```python
from build123d import *

# Parameters (mm, degrees)
SKETCH1_R           = 1.55
BOSS_EXTRUDE1_DEPTH = 5.8


with BuildPart() as part:
    # Sketch1 → Boss-Extrude1 (new body)
    with BuildSketch(Plane.XY):
        Polygon((-213.609090909, 31.65), (-213.609090909, 38.5), (-188.609090909, 38.5), (-188.609090909, 31.65), (-163.609090909, 31.65), (-163.609090909, 38.5), (-138.609090909, 38.5), (-138.609090909, 31.65), (-113.609090909, 31.65), (-113.609090909, 38.5), (-88.609090909, 38.5), (-88.609090909, 31.65), (-63.609090909, 31.65), (-63.609090909, 38.5), (-38.609090909, 38.5), (-38.609090909, 31.65), (-13.609090909, 31.65), (-13.609090909, 38.5), (11.390909091, 38.5), (11.390909091, 31.65), (36.390909091, 31.65), (36.390909091, 38.5), (61.390909091, 38.5), (61.390909091, 31.65), (86.390909091, 31.65), (86.390909091, 38.5), (111.390909091, 38.5), (111.390909091, 31.65), (136.390909091, 31.65), (136.390909091, 38.5), (161.390909091, 38.5), (161.390909091, 31.65), (186.390909091, 31.65), (186.390909091, 38.5), (211.390909091, 38.5), (211.390909091, 31.65), (236.390909091, 31.65), (236.390909091, 38.5), (261.390909091, 38.5), (261.390909091, 31.65), (274.040909091, 31.65), (274.040909091, 23.35), (283.890909091, 23.35), (283.890909091, 5.45), (274.040909091, 5.45), (274.040909091, -11.15), (283.890909091, -11.15), (283.890909091, -29.05), (274.040909091, -29.05), (274.040909091, -37.35), (261.390909091, -37.35), (261.390909091, -43.15), (236.390909091, -43.15), (236.390909091, -37.35), (211.390909091, -37.35), (211.390909091, -43.15), (186.390909091, -43.15), (186.390909091, -37.35), (161.390909091, -37.35), (161.390909091, -43.15), (136.390909091, -43.15), (136.390909091, -37.35), (111.390909091, -37.35), (111.390909091, -43.15), (86.390909091, -43.15), (86.390909091, -37.35), (61.390909091, -37.35), (61.390909091, -43.15), (36.390909091, -43.15), (36.390909091, -37.35), (11.390909091, -37.35), (11.390909091, -43.15), (-13.609090909, -43.15), (-13.609090909, -37.35), (-38.609090909, -37.35), (-38.609090909, -43.15), (-63.609090909, -43.15), (-63.609090909, -37.35), (-88.609090909, -37.35), (-88.609090909, -43.15), (-113.609090909, -43.15), (-113.609090909, -37.35), (-138.609090909, -37.35), (-138.609090909, -43.15), (-163.609090909, -43.15), (-163.609090909, -37.35), (-188.609090909, -37.35), (-188.609090909, -43.15), (-213.609090909, -43.15), (-213.609090909, -37.35), (-238.609090909, -37.35), (-238.609090909, -43.15), (-263.609090909, -43.15), (-263.609090909, -37.35), (-276.259090909, -37.35), (-276.259090909, -29.05), (-286.109090909, -29.05), (-286.109090909, -11.15), (-276.259090909, -11.15), (-276.259090909, 5.45), (-286.109090909, 5.45), (-286.109090909, 23.35), (-276.259090909, 23.35), (-276.259090909, 31.65), (-263.609090909, 31.65), (-263.609090909, 38.5), (-238.609090909, 38.5), (-238.609090909, 31.65), align=None)
        with Locations((-266.639090909, -20.1)):
            Circle(SKETCH1_R, mode=Mode.SUBTRACT)
        with Locations(Location((-266.639090909, 14.4, 0), (0, 0, 180))):
            Circle(SKETCH1_R, mode=Mode.SUBTRACT)
        with Locations((264.420909091, 14.4)):
            Circle(SKETCH1_R, mode=Mode.SUBTRACT)
        with Locations(Location((264.420909091, -20.1, 0), (0, 0, 180))):
            Circle(SKETCH1_R, mode=Mode.SUBTRACT)
        with Locations((-4.609090909, -27.73)):
            Circle(SKETCH1_R, mode=Mode.SUBTRACT)
        with Locations(Location((2.390909091, -27.73, 0), (0, 0, 180))):
            Circle(SKETCH1_R, mode=Mode.SUBTRACT)
        with Locations((175.390909091, -27.73)):
            Circle(SKETCH1_R, mode=Mode.SUBTRACT)
        with Locations(Location((182.390909091, -27.73, 0), (0, 0, 180))):
            Circle(SKETCH1_R, mode=Mode.SUBTRACT)
        with Locations((-184.609090909, -27.73)):
            Circle(SKETCH1_R, mode=Mode.SUBTRACT)
        with Locations(Location((-177.609090909, -27.73, 0), (0, 0, 180))):
            Circle(SKETCH1_R, mode=Mode.SUBTRACT)
    extrude(amount=BOSS_EXTRUDE1_DEPTH)


solid = part.part
```
The model under review builds one solid part; all positions refer to its coordinate system, in mm. Round coordinates to 2 decimals unless told otherwise and drop trailing zeros. Loops run counter-clockwise (first coordinate to the right, second up) from the corner with the lowest first, then second, coordinate; pieces in that order, holes last. Notation, with made-up numbers: (24.5, 44.5) -> (47.5, 44.5) arc R18 cw to (47.5, 72.5) -> close; hole circle Ø11 at (20, -10). An arc over 180 degrees is marked (long way). Answer as a JSON object with one key per item and string values. Group by question number.
1) We need section B-B on x = -78.5. Write out the cut boundary in (y, z).
2) We need section A-A on z = 3.15. Give the number of separate pieces and of enclosed holes in the cut face, then the cut area to 3 significant figures.
3) For line 1 (Y direction, x = 182.5, z = 3.7); line 2 (Y direction, x = 74, z = 0.35); line 3 (X direction, y = -10.5, z = 1.7), list the stretches that pass through material, from the lowest coordinate up. Write a range as [from, to].
4) For pin 1 Ø3 at (y, z) = (36, 3.5) entering from +X; pin 2 Ø3 at (y, z) = (-41, 3) entering from -X; pin 3 Ø2 at (y, z) = (-4.5, 3.5) entering from -X, all flat-tipped, find the tip position at first contact; note any pin that passes through.
Result set:
{
 "1": {"outline": "(-37.35, 0) -> (31.65, 0) -> (31.65, 5.8) -> (-37.35, 5.8) -> close"},
 "2": {"separate pieces": "1", "enclosed holes": "10", "area": "42,100 mm²"},
 "3": {"line 1": "[-37.35, -29.28], [-26.18, 31.65]", "line 2": "[-37.35, 31.65]", "line 3": "[-276.26, 274.04]"},
 "4": {"pin 1": "x = 261.39", "pin 2": "x = -263.61", "pin 3": "x = -276.26"}
}
